```python
from build123d import *

# Parameters (mm, degrees)
EXTRUDE_1_DEPTH     = 2
CUT_EXTRUDE_START   = -3
SKETCH_2_R          = 2
SKETCH_2_R_2        = 13
CUT_EXTRUDE_1_DEPTH = 3
CUT_EXTRUDE_START_2 = -10
CUT_EXTRUDE_2_DEPTH = 10
SKETCH_3_R          = 2.5
CUT_EXTRUDE_4_DEPTH = 10


with BuildPart() as part:
    # Sketch 1 → Extrude 1 (new body)
    with BuildSketch(Plane(origin=(0, 0, 0), x_dir=(0, 0, -1), z_dir=(1, 0, 0))):
        with BuildLine():
            Line((-105.367573178, 55.412145146), (-28.367573178, 55.412145146))
            ThreePointArc((-28.367573178, 55.412145146), (-7.367573178, 34.412145146), (-28.367573178, 13.412145146))
            Line((-28.367573178, 13.412145146), (-105.367573178, 13.412145146))
            Line((-105.367573178, 13.412145146), (-105.367573178, 55.412145146))
        make_face()
    extrude(amount=EXTRUDE_1_DEPTH)

    # Sketch 2 → Cut-Extrude 1 (cut)
    with BuildSketch(Plane(origin=(2, 0, 0), x_dir=(0, 0, -1), z_dir=(1, 0, 0)).offset(CUT_EXTRUDE_START)):
        with BuildLine():
            Line((-43.064511635, 19.412145146), (-108.765404369, 19.412145146))
            Line((-108.765404369, 19.412145146), (-108.765404369, 13.412145146))
            Line((-108.765404369, 13.412145146), (-28.367573178, 13.412145146))
            ThreePointArc((-28.367573178, 13.412145146), (-36.304827111, 14.96992305), (-43.064511635, 19.412145146))
        make_face()
        with Locations((-28.367573178, 51.912145146)):
            Circle(SKETCH_2_R)
        with Locations((-28.367573178, 16.912145146)):
            Circle(SKETCH_2_R)
        with Locations((-45.867573178, 34.412145146)):
            Circle(SKETCH_2_R)
        with Locations((-10.867573178, 34.412145146)):
            Circle(SKETCH_2_R)
        with Locations((-28.367573178, 34.412145146)):
            Circle(SKETCH_2_R_2)
    extrude(amount=CUT_EXTRUDE_1_DEPTH, mode=Mode.SUBTRACT)

    # Sketch 2_3 → Cut-Extrude 2 (cut)
    with BuildSketch(Plane(origin=(2, 0, 0), x_dir=(0, 0, -1), z_dir=(1, 0, 0)).offset(CUT_EXTRUDE_START_2)):
        with BuildLine():
            Line((-105.367573178, 55.412145146), (-105.367573178, 49.412145146))
            Line((-105.367573178, 49.412145146), (-43.064511635, 49.412145146))
            ThreePointArc((-43.064511635, 49.412145146), (-36.304827111, 53.854367241), (-28.367573178, 55.412145146))
            Line((-28.367573178, 55.412145146), (-105.367573178, 55.412145146))
        make_face()
    extrude(amount=CUT_EXTRUDE_2_DEPTH, mode=Mode.SUBTRACT)

    # Sketch 3 → Cut-Extrude 4 (cut)
    with BuildSketch(Plane(origin=(2, 0, 0), x_dir=(0, 0, -1), z_dir=(1, 0, 0))):
        with Locations((-97.867573178, 39.412145146)):
            Circle(SKETCH_3_R)
    extrude(amount=-CUT_EXTRUDE_4_DEPTH, mode=Mode.SUBTRACT)


solid = part.part
```
Could you check a few things on this model? Use its own coordinates, in mm. A direction names the side the tool comes from. Round coordinates to 2 decimals unless told otherwise and drop trailing zeros. Loops run counter-clockwise (first coordinate to the right, second up) from the corner with the lowest first, then second, coordinate; pieces in that order, holes last.
Q1. For P1, Ø1, axis at x = 1, y = 23, coming from the -Z side; P2, Ø4.5, axis at y = 39.41, z = 97.87, coming from the +X side; P3, Ø1, axis at y = 48, z = 36, coming from the -X side; P4, Ø1, axis at x = 0, y = 24, coming from the -Z side, each with a flat end and sliding along its axis, tell me the tip position at first contact or that it passes through.
Q2. I want a section at D-D (y = 40.5). Write out the boundary of the cut face in (x, z).
Q3. I want a section at A-A (x = 1.6). Write out the boundary of the cut face in (y, z), and give its area (3 significant figures).
Q4. I want a section at B-B (y = 16). Write out the boundary of the cut face in (x, z).
Q5. Thinking about a two-plate mould opening in Y: for faces 1 (the cylindrical face through (0.986, 17, 30.366)), 2 (the flat face through (1, 49.412, 75)), 3 (the flat face through (1, 34, 105.368)), which applies, pulls with the +Y half, pulls with the -Y half, needs draft (parallel to the pull), parting line crosses it, or undercut?
Q6. Please list where these lines run through material, in increasing order: L1, parallel to Z at x = 1.8, y = 29.5; L2, parallel to Z at x = 0.5, y = 35; L3, parallel to Z at x = 0.4, y = 43.5.
Q7. On a 3-axis mill with a long thin cutter (end or side, diameter ignored), from which of +Z, -Z, +X, -X, +Y, -Y can I reach the whole of each face in a straight line? I mean faces 4 (the cylindrical face through (0.986, 33.195, 47.455)), 5 (the flat face through (1, 19.412, 74)). Say none if no direction works.
Q8. I want a section at C-C (z = 39). Write out the boundary of the cut face in (x, y), and give its area (3 significant figures).
Answer below:
1. P1: stops at z = 10.43
1. P2: passes through
1. P3: stops at x = 0
1. P4: stops at z = 9.85
2. outline: (0, 8.27) - (2, 8.27) - (2, 16.88) - (0, 16.88) - close; (0, 39.85) - (2, 39.85) - (2, 95.62) - (0, 95.62) - close; (0, 100.12) - (2, 100.12) - (2, 105.37) - (0, 105.37) - close
3. outline: (19.41, 43.06) arc R21 ccw (long way) to (49.41, 43.06) - (49.41, 105.37) - (19.41, 105.37) - close; hole circle Ø4 at (16.91, 28.37); hole circle Ø26 at (34.41, 28.37); hole circle Ø4 at (34.41, 10.87); hole circle Ø4 at (34.41, 45.87); hole circle Ø5 at (39.41, 97.87); hole circle Ø4 at (51.91, 28.37)
3. area: 2,520 mm2
4. outline: (0, 18.27) - (2, 18.27) - (2, 26.59) - (0, 26.59) - close; (0, 30.15) - (2, 30.15) - (2, 38.47) - (0, 38.47) - close
5. face 1: undercut
5. face 2: pulls with the +Y half
5. face 3: needs draft
6. L1: z = 7.95 to 16.33, 40.4 to 105.37
6. L2: z = 7.38 to 8.96, 12.78 to 15.38, 41.35 to 43.96, 47.78 to 105.37
6. L3: z = 9.44 to 19.07, 37.66 to 105.37
7. face 4: +X, -X
7. face 5: +Z, +X, -X, -Y
8. outline: (0, 16.3) - (2, 16.3) - (2, 26.93) - (0, 26.93) - close; (0, 41.89) - (2, 41.89) - (2, 52.52) - (0, 52.52) - close
8. area: 42.5 mm2
